```python
from build123d import *

# Parameters (mm, degrees)
F0_W     = 18.161
F0_H     = 14.732
F1_DEPTH = 12.7
F2_W     = 14.732
F2_H     = 10.668
F3_DEPTH = 4.318
F4_W     = 1.016
F4_H     = 1.016
F5_DEPTH = 5.08


with BuildPart() as f1:
    # F0 (on Top) → F1 (new body)
    with BuildSketch(Plane.XY):
        Rectangle(F0_W, F0_H)
    extrude(amount=F1_DEPTH)

    # F2 (on face) → F3 (join)
    with BuildSketch(Plane(origin=(0, 0, 0), x_dir=(1, 0, 0), z_dir=(0, 0, -1))):
        with Locations((0, -2.032)):
            Rectangle(F2_W, F2_H)
    extrude(amount=F3_DEPTH)

    # F4 (on face) → F5 (join)
    with BuildSketch(Plane(origin=(0, 0, 0), x_dir=(1, 0, 0), z_dir=(0, 0, -1))):
        with Locations((-7.49935, 6.096)):
            Rectangle(F4_W, F4_H)
        with Locations((-2.49936, 6.096)):
            Rectangle(F4_W, F4_H)
        with Locations((2.49936, 6.096)):
            Rectangle(F4_W, F4_H)
        with Locations((7.49935, 6.096)):
            Rectangle(F4_W, F4_H)
    extrude(amount=F5_DEPTH)


solid = f1.part
```
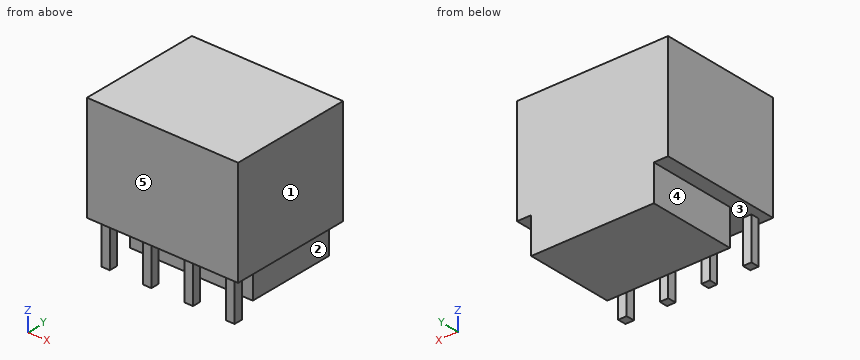
Geometry: final body of the model. Coordinates: model frame, mm. Face numbers are marked on the shaded views. A direction names the side the tool comes from. Coordinates: 2 decimals unless noted, no trailing zeros. Order: outer loops, then holes, each group sorted by start corner. A loop starts at its lowest first (then second) coordinate and runs counter-clockwise, first axis right, second up. Notation, with made-up numbers: (82.25, 76) -> (130.25, 76) arc R31 cw to (130.25, 102) -> close; hole circle Ø1 at (-17.5, 58.25). An arc over 180 degrees is marked (long way). Write item = value, one per line.
(1) Line query: line 1 (Y direction, x = 2.25, z = -2); line 2 (Z direction, x = -2.75, y = 0.75); line 3 (Z direction, x = 7.5, y = -5). Output: solid intervals per line, ascending.
Solved:
line_1 = -6.6 to -5.59, -3.3 to 7.37
line_2 = -4.32 to 12.7
line_3 = 0 to 12.7
(2) Access query for the marked faces 1 and 2. Directions: +Z, -Z, +X, -X, +Y, -Y. A direction counts if a zero-diameter tool reaches every point of the face in a straight line with its end or side. Return the directions, or none.
Solved:
face_1 = +Z, -Z, +X, +Y, -Y
face_2 = -Z, +X, +Y
(3) Pull-direction query (X, two-part tool) for the marked faces 3, 4 and 5; classes: pulls with the +X half, pulls with the -X half, needs draft (parallel to the pull), parting line crosses it, or undercut.
Solved:
face_3 = undercut
face_4 = pulls with the -X half
face_5 = needs draft
(4) Cut plane B-B on x = 3.5. Return loops of the section in (y, z), plus the area to 3 significant figures.
Solved:
outline = (-7.37, 0) -> (-3.3, 0) -> (-3.3, -4.32) -> (7.37, -4.32) -> (7.37, 12.7) -> (-7.37, 12.7) -> close
area = 233 mm²
(5) Cut plane C-C on y = -5.25. Return loops of the section in (x, z).
Solved:
outline = (-9.08, 0) -> (9.08, 0) -> (9.08, 12.7) -> (-9.08, 12.7) -> close
(6) Pin query (flat end, axial travel): pin 1 Ø0.8 at (x, z) = (-7.5, -3.5) entering from -Y; pin 2 Ø0.8 at (y, z) = (-6, -3.5) entering from -X; pin 3 Ø1.3 at (y, z) = (-0.5, -1.5) entering from +X. Return the tip coordinate at first contact, or that it passes through.
Solved:
pin_1 = -6.6
pin_2 = -8.01
pin_3 = 7.37
(7) Cut plane A-A on y = 3.25. Return loops of the section in (x, z), plus the area to 3 significant figures.
Solved:
outline = (-9.08, 0) -> (-7.37, 0) -> (-7.37, -4.32) -> (7.37, -4.32) -> (7.37, 0) -> (9.08, 0) -> (9.08, 12.7) -> (-9.08, 12.7) -> close
area = 294 mm²
